Part print with two shaded views. Sizes in mm from the minimum x, y, z corner. Round coordinates to 2 decimals unless told otherwise and drop trailing zeros. Write each loop counter-clockwise with the first axis right and the second up, starting at its lowest first coordinate (ties: lowest second). Pieces come first, ordered by that corner, then holes. Notation, with made-up numbers: (-13, 44.25) -> (17, 44.25) arc R16 cw to (17, 52.25) -> close; hole circle Ø9 at (43.5, 57). An arc over 180 degrees is marked (long way). Answer in a Markdown table with one row per item. Add a question column.
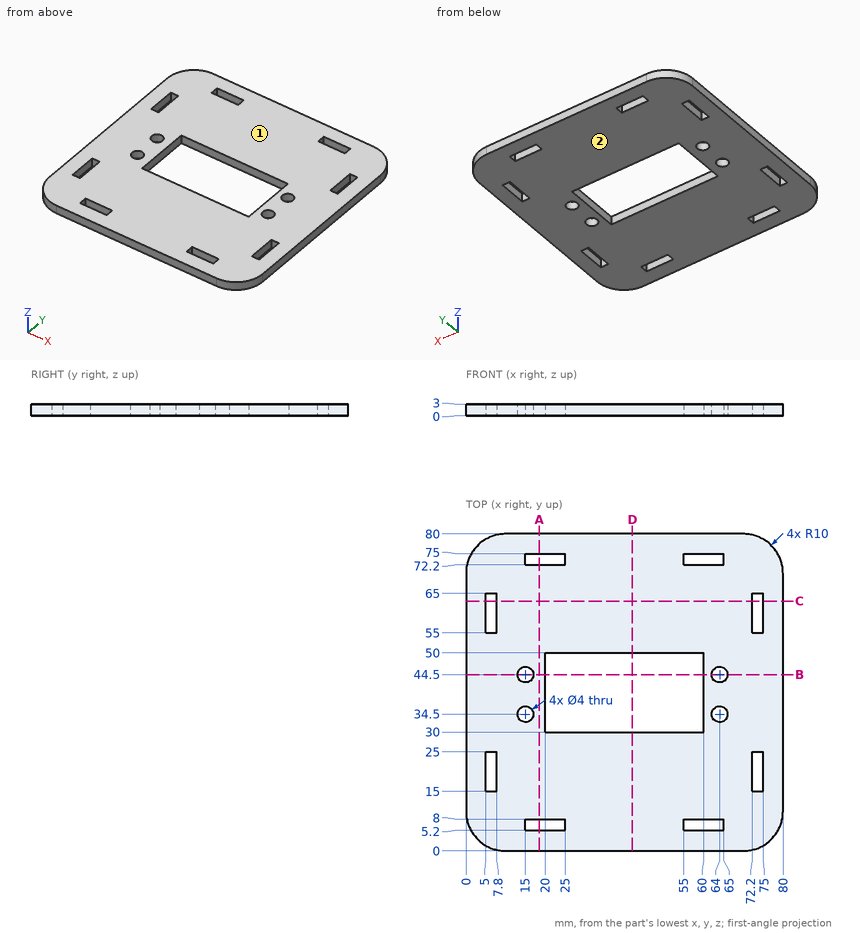
Item 1: Saw through at C-C on y = 63. Give the cut face in (x, z).
Item 2: Two-plate mould, pull along Z, no slides. Class the marked faces 1 and 2: +Z half, -Z half, draft (parallel to the pull), parting line (faces both ways), or undercut.
Item 3: Saw through at B-B on y = 44.5. Give the cut face in (x, z).
Item 4: Pin check, flat tips, straight feed: pin 1 (2.5 mm diameter, centred on x = 64, y = 44.5, fed in from -Z); pin 2 (1.4 mm diameter, centred on x = 6, z = 2, fed in from -Y). Stop position of each tip, or through.
Item 5: Drill centre lines: probe 1 along Y at (x, z) = (59, 0.45); probe 2 along Y at (x, z) = (64, 0.7); probe 3 along X at (y, z) = (49.5, 2.2). Where is each one in solid material? Low to high.
Item 6: Saw through at A-A on x = 18.5. Give the cut face in (y, z), then the cut area to 3 significant figures.
Item 7: Saw through at D-D on x = 42. Give the cut face in (y, z), then the cut area to 3 significant figures.
Recorded:
| question | item | result |
|---|---|---|
| 1 | outline | (0, 0) -> (5, 0) -> (5, 3) -> (0, 3) -> close; (7.8, 0) -> (72.2, 0) -> (72.2, 3) -> (7.8, 3) -> close; (75, 0) -> (80, 0) -> (80, 3) -> (75, 3) -> close |
| 2 | face 1 | +Z half |
| 2 | face 2 | -Z half |
| 3 | outline | (0, 0) -> (13, 0) -> (13, 3) -> (0, 3) -> close; (17, 0) -> (20, 0) -> (20, 3) -> (17, 3) -> close; (60, 0) -> (62, 0) -> (62, 3) -> (60, 3) -> close; (66, 0) -> (80, 0) -> (80, 3) -> (66, 3) -> close |
| 4 | pin 1 | through |
| 4 | pin 2 | y = 0.56 |
| 5 | probe 1 | 0 to 5.2, 8 to 30, 50 to 72.2, 75 to 80 |
| 5 | probe 2 | 0 to 5.2, 8 to 32.5, 36.5 to 42.5, 46.5 to 72.2, 75 to 80 |
| 5 | probe 3 | 0 to 20, 60 to 80 |
| 6 | outline | (0, 0) -> (5.2, 0) -> (5.2, 3) -> (0, 3) -> close; (8, 0) -> (72.2, 0) -> (72.2, 3) -> (8, 3) -> close; (75, 0) -> (80, 0) -> (80, 3) -> (75, 3) -> close |
| 6 | area | 223 mm2 |
| 7 | outline | (0, 0) -> (30, 0) -> (30, 3) -> (0, 3) -> close; (50, 0) -> (80, 0) -> (80, 3) -> (50, 3) -> close |
| 7 | area | 180 mm2 |
